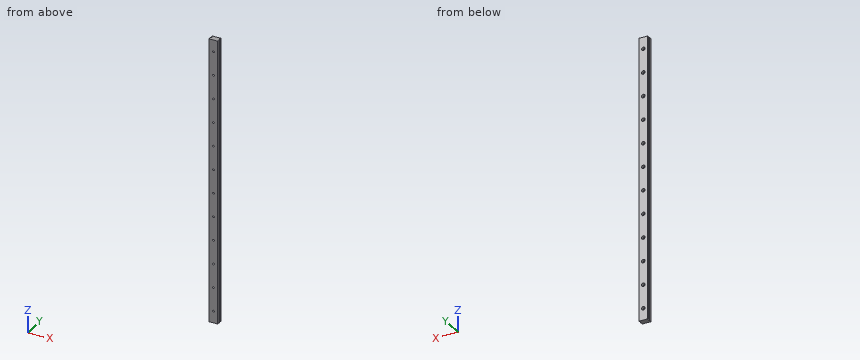
```python
from build123d import *

# Parameters (mm, degrees)
EXTRUDE_1_DEPTH        = 1000
SKETCH_2_R             = 1.5
CUT_EXTRUDE_1_DEPTH    = 20
SKETCH_3_R             = 3
CUT_EXTRUDE_2_DEPTH    = 4.5
PATTERN_LINEAR_1_COUNT = 25
PATTERN_LINEAR_1_PITCH = 40
CUT_EXTRUDE_4_DEPTH    = 80
CUT_EXTRUDE_5_DEPTH    = 80
CUT_EXTRUDE_START      = -360
CUT_EXTRUDE_7_DEPTH    = 360


with BuildPart() as part:
    # 草图1 → 凸台-拉伸1 (new body)
    with BuildSketch(Plane.XY):
        with BuildLine():
            Line((-7.643186957, 0.234233912), (-7.643186957, -4.365766088))
            Line((-7.643186957, -4.365766088), (-7.243186957, -4.765766088))
            Line((-7.243186957, -4.765766088), (6.956813043, -4.765766088))
            Line((6.956813043, -4.765766088), (7.356813043, -4.365766088))
            Line((7.356813043, -4.365766088), (7.356813043, 0.234233912))
            ThreePointArc((7.356813043, 0.234233912), (6.296152871, 0.67357374), (5.856813043, 1.734233912))
            ThreePointArc((5.856813043, 1.734233912), (6.296152871, 2.794894084), (7.356813043, 3.234233912))
            Line((7.356813043, 3.234233912), (7.356813043, 4.834233912))
            Line((7.356813043, 4.834233912), (6.956813043, 5.234233912))
            Line((6.956813043, 5.234233912), (-7.243186957, 5.234233912))
            Line((-7.243186957, 5.234233912), (-7.643186957, 4.834233912))
            Line((-7.643186957, 4.834233912), (-7.643186957, 3.234233912))
            ThreePointArc((-7.643186957, 3.234233912), (-6.143186957, 1.734233912), (-7.643186957, 0.234233912))
        make_face()
    extrude(amount=EXTRUDE_1_DEPTH)

    # 草图2 → 切除-拉伸1 (cut)
    with BuildSketch(Plane(origin=(0, 5.234233912, 0), x_dir=(1, 0, 0), z_dir=(0, 1, 0))):
        with Locations(Location((0, -20, 0), (0, 0, 270))):
            Circle(SKETCH_2_R)
    cut_extrude_1 = extrude(amount=-CUT_EXTRUDE_1_DEPTH, mode=Mode.SUBTRACT)

    # 草图3 → 切除-拉伸2 (cut)
    with BuildSketch(Plane(origin=(0, 5.234233912, 0), x_dir=(1, 0, 0), z_dir=(0, 1, 0))):
        with Locations(Location((0, -20, 0), (0, 0, 270))):
            Circle(SKETCH_3_R)
    cut_extrude_2 = extrude(amount=-CUT_EXTRUDE_2_DEPTH, mode=Mode.SUBTRACT)

    # 阵列(线性)1: 切除-拉伸1, 切除-拉伸2 ×25
    with Locations(*[(0, 0, i * PATTERN_LINEAR_1_PITCH) for i in range(1, PATTERN_LINEAR_1_COUNT)]):
        add(cut_extrude_1, mode=Mode.SUBTRACT)
        add(cut_extrude_2, mode=Mode.SUBTRACT)

    # 草图6 → 切除-拉伸4 (cut)
    with BuildSketch(Plane(origin=(0, 0, 0), x_dir=(-1, 0, 0), z_dir=(0, 0, -1))):
        with BuildLine():
            Line((7.643186957, 3.234233912), (7.643186957, 4.834233912))
            Line((7.643186957, 4.834233912), (7.243186957, 5.234233912))
            Line((7.243186957, 5.234233912), (-6.956813043, 5.234233912))
            Line((-6.956813043, 5.234233912), (-7.356813043, 4.834233912))
            Line((-7.356813043, 4.834233912), (-7.356813043, 3.234233912))
            ThreePointArc((-7.356813043, 3.234233912), (-5.856813043, 1.734233912), (-7.356813043, 0.234233912))
            Line((-7.356813043, 0.234233912), (-7.356813043, -4.365766088))
            Line((-7.356813043, -4.365766088), (-6.956813043, -4.765766088))
            Line((-6.956813043, -4.765766088), (7.243186957, -4.765766088))
            Line((7.243186957, -4.765766088), (7.643186957, -4.365766088))
            Line((7.643186957, -4.365766088), (7.643186957, 0.234233912))
            ThreePointArc((7.643186957, 0.234233912), (6.143186957, 1.734233912), (7.643186957, 3.234233912))
        make_face()
    extrude(amount=-CUT_EXTRUDE_4_DEPTH, mode=Mode.SUBTRACT)

    # 草图7 → 切除-拉伸5 (cut)
    with BuildSketch(Plane(origin=(0, 0, 80), x_dir=(-1, 0, 0), z_dir=(0, 0, -1))):
        with BuildLine():
            Line((7.643186957, 3.234233912), (7.643186957, 4.834233912))
            Line((7.643186957, 4.834233912), (7.243186957, 5.234233912))
            Line((7.243186957, 5.234233912), (-6.956813043, 5.234233912))
            Line((-6.956813043, 5.234233912), (-7.356813043, 4.834233912))
            Line((-7.356813043, 4.834233912), (-7.356813043, 3.234233912))
            ThreePointArc((-7.356813043, 3.234233912), (-5.856813043, 1.734233912), (-7.356813043, 0.234233912))
            Line((-7.356813043, 0.234233912), (-7.356813043, -4.365766088))
            Line((-7.356813043, -4.365766088), (-6.956813043, -4.765766088))
            Line((-6.956813043, -4.765766088), (7.243186957, -4.765766088))
            Line((7.243186957, -4.765766088), (7.643186957, -4.365766088))
            Line((7.643186957, -4.365766088), (7.643186957, 0.234233912))
            ThreePointArc((7.643186957, 0.234233912), (6.143186957, 1.734233912), (7.643186957, 3.234233912))
        make_face()
    extrude(amount=-CUT_EXTRUDE_5_DEPTH, mode=Mode.SUBTRACT)

    # 草图9 → 切除-拉伸7 (cut)
    with BuildSketch(Plane.XY.offset(1000).offset(CUT_EXTRUDE_START)):
        with BuildLine():
            Line((-7.643186957, 0.234233912), (-7.643186957, -4.365766088))
            Line((-7.643186957, -4.365766088), (-7.243186957, -4.765766088))
            Line((-7.243186957, -4.765766088), (6.956813043, -4.765766088))
            Line((6.956813043, -4.765766088), (7.356813043, -4.365766088))
            Line((7.356813043, -4.365766088), (7.356813043, 0.234233912))
            ThreePointArc((7.356813043, 0.234233912), (5.856813043, 1.734233912), (7.356813043, 3.234233912))
            Line((7.356813043, 3.234233912), (7.356813043, 4.834233912))
            Line((7.356813043, 4.834233912), (6.956813043, 5.234233912))
            Line((6.956813043, 5.234233912), (-7.243186957, 5.234233912))
            Line((-7.243186957, 5.234233912), (-7.643186957, 4.834233912))
            Line((-7.643186957, 4.834233912), (-7.643186957, 3.234233912))
            ThreePointArc((-7.643186957, 3.234233912), (-6.143186957, 1.734233912), (-7.643186957, 0.234233912))
        make_face()
    extrude(amount=CUT_EXTRUDE_7_DEPTH, mode=Mode.SUBTRACT)


solid = part.part
```
The listing builds one solid part. Answer for the finished solid, in the listing's coordinates (mm). Give positions to 0.01 mm unless a question says otherwise; leave off trailing zeros. Order: outer loops, then holes, each group sorted by start corner. A loop starts at its lowest first (then second) coordinate and runs counter-clockwise, first axis right, second up. Notation, with made-up numbers: (47, 22) - (59, 22) arc R13 ccw to (59, 33) - close; hole circle Ø9 at (69, 27.25). An arc over 180 degrees is marked (long way). Answer in a Markdown table with one row per item. Add a question column.
Q1. Find the intervals of material crossed by line 1 along X through (y, z) = (3.7, 380); line 2 along Y through (x, z) = (1.75, 222); line 3 along X through (y, z) = (2.6, 300), in increasing order. Write a range as [from, to].
Q2. Given P1, Ø5, axis at x = 0, z = 260, coming from the -Y side; P2, Ø5.5, axis at x = 0, z = 420, coming from the +Y side, each flat-ended and moving along its own axis, determine where each tip first touches the part or whether it passes through.
Q3. The part is cut by section A-A (z = 323). Determine the outline of the cut face in (x, y).
Determined:
| question | item | result |
|---|---|---|
| 1 | line 1 | x = [-7.64, -3], [3, 7.36] |
| 1 | line 2 | y = [-4.77, 0.73] |
| 1 | line 3 | x = [-6.42, -3], [3, 6.13] |
| 2 | P1 | stops at y = -4.77 |
| 2 | P2 | stops at y = 0.73 |
| 3 | outline | (-7.64, -4.37) - (-7.24, -4.77) - (6.96, -4.77) - (7.36, -4.37) - (7.36, 0.23) arc R1.5 cw to (7.36, 3.23) - (7.36, 4.83) - (6.96, 5.23) - (-7.24, 5.23) - (-7.64, 4.83) - (-7.64, 3.23) arc R1.5 cw to (-7.64, 0.23) - close |
